Read the model definition and answer for the solid it produces. Units are mm, in the model's axes. Face numbers are marked on the shaded views. Coordinates: 2 decimals unless noted, no trailing zeros. Order: outer loops, then holes, each group sorted by start corner. A loop starts at its lowest first (then second) coordinate and runs counter-clockwise, first axis right, second up. Notation, with made-up numbers: (82, 17) -> (109, 17) arc R26 ccw to (109, 35) -> close; hole circle Ø8 at (9, -37). An arc over 180 degrees is marked (long way). Answer in a Markdown table with one row per item.
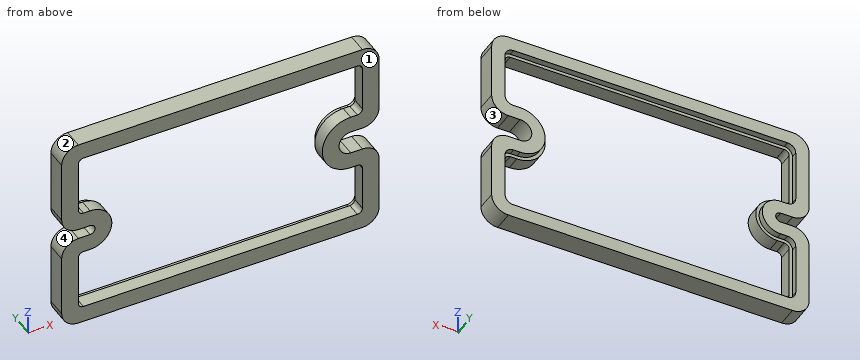
from build123d import *

# Parameters (mm, degrees)
SKETCH1_W           = 95
SKETCH1_H           = 60
BOSS_EXTRUDE1_DEPTH = 6
SKETCH6_R           = 3.5
SKETCH6_R_2         = 1.5
CUT_EXTRUDE3_DEPTH  = 113.521109131
CUT_EXTRUDE1_DEPTH  = 113.521109131
FILLET3_R           = 1.5
SKETCH7_W           = 8.5
SKETCH7_H           = 3
SKETCH7_H_2         = 7
CUT_EXTRUDE4_DEPTH  = 113.521109131
FILLET4_R           = 5
FILLET5_R           = 1.5
CUT_EXTRUDE5_DEPTH  = 1.8


with BuildPart() as part:
    # Sketch1 → Boss-Extrude1 (new body)
    with BuildSketch(Plane(origin=(0, 0, 0), x_dir=(1, 0, 0), z_dir=(0, 1, 0))):
        with Locations((47.5, 30)):
            Rectangle(SKETCH1_W, SKETCH1_H)
    extrude(amount=BOSS_EXTRUDE1_DEPTH)

    # Sketch6 → Cut-Extrude3 (cut, through all)
    with BuildSketch(Plane.XZ):
        with Locations(Location((86.5, -30, 0), (0, 0, 270))):
            Circle(SKETCH6_R)
        with Locations(Location((8.5, -30, 0), (0, 0, 270))):
            Circle(SKETCH6_R_2)
    extrude(amount=-CUT_EXTRUDE3_DEPTH, mode=Mode.SUBTRACT)

    # Sketch2 → Cut-Extrude1 (cut, through all)
    with BuildSketch(Plane(origin=(0, 6, 0), x_dir=(-1, 0, 0), z_dir=(0, 1, 0))):
        with BuildLine():
            Line((-8.5, -36.5), (-5, -36.5))
            Line((-5, -36.5), (-5, -55))
            Line((-5, -55), (-90, -55))
            Line((-90, -55), (-90, -38.5))
            Line((-90, -38.5), (-86.5, -38.5))
            ThreePointArc((-86.5, -38.5), (-78, -30), (-86.5, -21.5))
            Line((-86.5, -21.5), (-90, -21.5))
            Line((-90, -21.5), (-90, -5))
            Line((-90, -5), (-5, -5))
            Line((-5, -5), (-5, -23.5))
            Line((-5, -23.5), (-8.5, -23.5))
            ThreePointArc((-8.5, -23.5), (-15, -30), (-8.5, -36.5))
        make_face()
    extrude(amount=-CUT_EXTRUDE1_DEPTH, mode=Mode.SUBTRACT)

    # Fillet3
    fillet3_edges = [part.edges().sort_by_distance(p)[0] for p in [
        (90, 3, -55),
    ]]
    fillet(fillet3_edges, radius=FILLET3_R)

    # Sketch7 → Cut-Extrude4 (cut, through all)
    with BuildSketch(Plane(origin=(0, 6, 0), x_dir=(-1, 0, 0), z_dir=(0, 1, 0))):
        with Locations((-4.25, -30)):
            Rectangle(SKETCH7_W, SKETCH7_H)
        with Locations((-90.75, -30)):
            Rectangle(SKETCH7_W, SKETCH7_H_2)
    extrude(amount=-CUT_EXTRUDE4_DEPTH, mode=Mode.SUBTRACT)

    # Fillet4
    fillet4_edges = [part.edges().sort_by_distance(p)[0] for p in [
        (0, 3, -60),
        (95, 3, -60),
        (0, 3, -28.5),
        (95, 3, 0),
        (0, 3, -31.5),
        (0, 3, 0),
        (95, 3, -33.5),
        (95, 3, -26.5),
    ]]
    fillet(fillet4_edges, radius=FILLET4_R)

    # Fillet5
    fillet5_edges = [part.edges().sort_by_distance(p)[0] for p in [
        (5, 3, -5),
        (5, 3, -23.5),
        (5, 3, -36.5),
        (5, 3, -55),
        (90, 3, -38.5),
        (90, 3, -21.5),
        (90, 3, -5),
    ]]
    fillet(fillet5_edges, radius=FILLET5_R)

    # Sketch9 → Cut-Extrude5 (cut)
    with BuildSketch(Plane(origin=(0, 6, 0), x_dir=(1, 0, 0), z_dir=(0, 1, 0))):
        with BuildLine():
            Line((6.5, 4), (88.5, 4))
            ThreePointArc((88.5, 4), (90.267766953, 4.732233047), (91, 6.5))
            Line((91, 6.5), (91, 20))
            ThreePointArc((91, 20), (90.267766953, 21.767766953), (88.5, 22.5))
            Line((88.5, 22.5), (86.5, 22.5))
            ThreePointArc((86.5, 22.5), (79, 30), (86.5, 37.5))
            Line((86.5, 37.5), (88.5, 37.5))
            ThreePointArc((88.5, 37.5), (90.267766953, 38.232233047), (91, 40))
            Line((91, 40), (91, 53.5))
            ThreePointArc((91, 53.5), (90.267766953, 55.267766953), (88.5, 56))
            Line((88.5, 56), (6.5, 56))
            ThreePointArc((6.5, 56), (4.732233047, 55.267766953), (4, 53.5))
            Line((4, 53.5), (4, 38))
            ThreePointArc((4, 38), (4.732233047, 36.232233047), (6.5, 35.5))
            Line((6.5, 35.5), (8.5, 35.5))
            ThreePointArc((8.5, 35.5), (14, 30), (8.5, 24.5))
            Line((8.5, 24.5), (6.5, 24.5))
            ThreePointArc((6.5, 24.5), (4.732233047, 23.767766953), (4, 22))
            Line((4, 22), (4, 6.5))
            ThreePointArc((4, 6.5), (4.732233047, 4.732233047), (6.5, 4))
        make_face()
    extrude(amount=-CUT_EXTRUDE5_DEPTH, mode=Mode.SUBTRACT)


solid = part.part
Q1. The part is cut by section B-B (x = 52). Write down the section's boundary in (y, z).
Outcome:
| item | result |
|---|---|
| outline | (0, -60) -> (6, -60) -> (6, -56) -> (4.2, -56) -> (4.2, -55) -> (0, -55) -> close; (0, -5) -> (4.2, -5) -> (4.2, -4) -> (6, -4) -> (6, 0) -> (0, 0) -> close |
Q2. The part is cut by section A-A (z = -30). Write down the section's boundary in (x, y), then the cut area to 3 significant figures.
Outcome:
| item | result |
|---|---|
| outline | (10, 0) -> (15, 0) -> (15, 4.2) -> (14, 4.2) -> (14, 6) -> (10, 6) -> close; (78, 0) -> (83, 0) -> (83, 6) -> (79, 6) -> (79, 4.2) -> (78, 4.2) -> close |
| area | 56.4 mm² |
Q3. Consider line 1 (X direction, y = 2.2, z = -49); line 2 (Z direction, x = 62, y = 5.55); line 3 (Z direction, x = 36.5, y = 2.6). Determine where each line is inside the solid, lowest interval first.
Outcome:
| item | result |
|---|---|
| line 1 | 0 to 5, 90 to 95 |
| line 2 | -60 to -56, -4 to 0 |
| line 3 | -60 to -55, -5 to 0 |
Q4. For a pull along Z with two mould halves and no side action, classify the marked faces 1, 2, 3 and 4 as pulls with the +Z half, pulls with the -Z half, needs draft (parallel to the pull), parting line crosses it, or undercut.
Outcome:
| item | result |
|---|---|
| face 1 | needs draft |
| face 2 | pulls with the +Z half |
| face 3 | undercut |
| face 4 | undercut |
